Verification items for the finished model (mm, model axes). Face numbers are marked on the shaded views. A direction names the side the tool comes from. Round coordinates to 2 decimals unless told otherwise and drop trailing zeros. Loops run counter-clockwise (first coordinate to the right, second up) from the corner with the lowest first, then second, coordinate; pieces in that order, holes last. Notation, with made-up numbers: M 82,-17.5 L 137,-17.5 A22 cw 137,19.5 Z; hole C 29.5,15.5 d6. An arc over 180 degrees is marked long. Answer as CSV lines item,"result".
```python
from build123d import *

# Parameters (mm, degrees)
SKETCH3_R           = 1.7145000000000004
SKETCH3_R_2         = 1.7144999999999995
BOSS_EXTRUDE1_DEPTH = 3.175
BOSS_EXTRUDE2_DEPTH = 36.83
LPATTERN2_COUNT     = 2
LPATTERN2_PITCH     = 9.525
CUT_EXTRUDE1_DEPTH  = 54.24920844482103
FILLET1_R           = 3.175


with BuildPart() as part:
    # Sketch3 → Boss-Extrude1 (new body)
    with BuildSketch(Plane.XY):
        with BuildLine():
            ThreePointArc((23.718196461855243, 14.429078391112267), (20.955, 15.061802351494215), (18.191803538144754, 14.429078391112267))
            Line((18.191803538144754, 14.429078391112265), (-2.009608404339229, 4.6656054335111925))
            Line((-2.009608404339229, 4.6656054335111925), (-2.407325349839823, 4.473386263225946))
            ThreePointArc((-2.4073253498398226, 4.473386263225944), (-4.1812606420695575, -2.885040631096911), (3.3277025000445404, -3.83833245970139))
            Line((3.3277025000445413, -3.8383324597013875), (17.32713374877397, 5.9068077182607865))
            ThreePointArc((17.32713374877397, 5.9068077182607865), (20.955, 7.045177794406333), (24.58286625122603, 5.90680771826079))
            Line((24.58286625122603, 5.906807718260788), (38.58229749995545, -3.838332459701375))
            ThreePointArc((38.58229749995546, -3.8383324597013706), (46.09126064206956, -2.8850406310969055), (44.31732534983981, 4.4733862632259465))
            Line((44.31732534983981, 4.473386263225951), (43.91960840433945, 4.665605433511086))
            Line((43.91960840433945, 4.665605433511086), (23.718196461855243, 14.429078391112267))
        make_face()
        Circle(SKETCH3_R, mode=Mode.SUBTRACT)
        with Locations((41.91, 0)):
            Circle(SKETCH3_R_2, mode=Mode.SUBTRACT)
    boss_extrude1 = extrude(amount=BOSS_EXTRUDE1_DEPTH)

    # Sketch4 → Boss-Extrude2 (add)
    with BuildSketch(Plane(origin=(0, 15.239999999999998, 0), x_dir=(1, 0, 0), z_dir=(0, 1, 0))):
        Polygon((11.43, 0), (30.480000000000004, 2.33e-15), (30.48, 6.350000000000002), (11.43, 6.35), align=None)
    extrude(amount=-BOSS_EXTRUDE2_DEPTH)

    # LPattern2: Boss-Extrude1 ×2
    with Locations(*[(0, 0, -i * LPATTERN2_PITCH) for i in range(1, LPATTERN2_COUNT)]):
        add(boss_extrude1)

    # Sketch5 → Cut-Extrude1 (cut, through all)
    with BuildSketch(Plane.XY.offset(3.175)):
        with BuildLine():
            Line((36.195, 8.398958601029964), (23.718196461855243, 14.429078391112268))
            ThreePointArc((23.718196461855243, 14.429078391112268), (20.955, 15.061802351494219), (18.191803538144754, 14.429078391112267))
            Line((18.191803538144754, 14.429078391112267), (5.715000000000005, 8.39895860102995))
            Line((5.715000000000005, 8.39895860102995), (5.714999999999998, 15.239999999999984))
            Line((5.714999999999998, 15.239999999999984), (36.195, 15.239999999999998))
            Line((36.195, 15.239999999999998), (36.195, 8.398958601029964))
        make_face()
        with BuildLine():
            Line((30.480000000000004, 1.8017555908602794), (24.58286625122603, 5.906807718260787))
            ThreePointArc((24.58286625122603, 5.906807718260787), (20.955000000000002, 7.045177794406331), (17.327133748773974, 5.906807718260784))
            Line((17.327133748773974, 5.906807718260784), (11.430000000000003, 1.8017555908602725))
            Line((11.430000000000003, 1.8017555908602725), (11.430000000000026, -23.117342691118424))
            Line((11.430000000000026, -23.117342691118424), (30.480000000000004, -23.117342691118413))
            Line((30.480000000000004, -23.117342691118413), (30.480000000000004, 1.8017555908602794))
        make_face()
    extrude(amount=-CUT_EXTRUDE1_DEPTH, mode=Mode.SUBTRACT)

    # Fillet1
    fillet1_edges = [part.edges().sort_by_distance(p)[0] for p in [
        (30.480000000000004, 1.8017555908602794, -3.1750000000000016),
        (11.430000000000003, 1.8017555908602725, -3.175),
        (30.48, 11.161055038227271, -3.1750000000000016),
        (11.43, 11.16105503822726, -3.1749999999999994),
    ]]
    fillet(fillet1_edges, radius=FILLET1_R)


solid = part.part
```
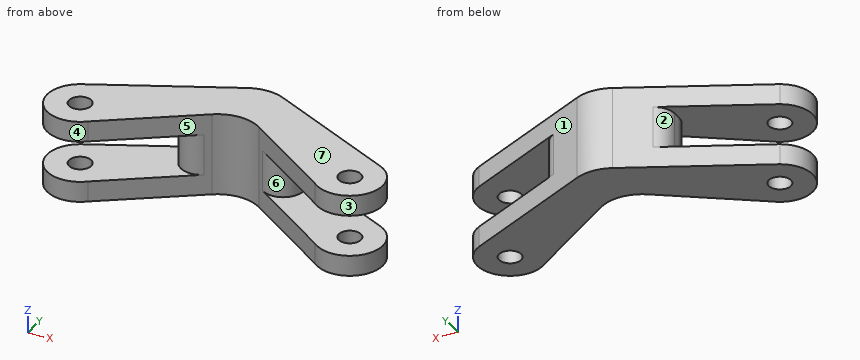
1) Section check B-B (z = -8.5). State how many separate pieces and enclosed holes the cut face has, plus the area to 3 significant figures.
Here are the results:
separate pieces,"1"
enclosed holes,"2"
area,"464 mm^2"
2) Material ranges on probe 1 along Z at (x, y) = (30.5, 5.75) (3 decimals); probe 2 along X at (y, z) = (6.5, -2.75); probe 3 along X at (y, z) = (9.75, -7.25), recorded low to high.
Here are the results:
probe 1,"z = -9.525 to -6.35, 0 to 3.175"
probe 2,"x = 11.75 to 18.38, 23.53 to 30.16"
probe 3,"x = 8.51 to 33.4"
3) Draft check along X on the marked faces 1, 2, 3 and 4. Enter one of: +X half, -X half, draft (parallel to the pull), parting line (faces both ways), or undercut.
Here are the results:
face 1,"+X half"
face 2,"-X half"
face 3,"undercut"
face 4,"undercut"
4) Go/stop test with flat-tipped pins: pin 1 (5.5 mm diameter, centred on x = 41.91, y = 0, fed in from -Z) (3 decimals); pin 2 (2 mm diameter, centred on x = 0, y = 0, fed in from +Z); pin 3 (1 mm diameter, centred on y = 8.5, z = -4.5, fed in from +X); pin 4 (5 mm diameter, centred on y = 8.5, z = 0, fed in from -X). Record where each tip stops, or that it passes through.
Here are the results:
pin 1,"stops at z = -9.525"
pin 2,"passes through"
pin 3,"stops at x = 30.48"
pin 4,"stops at x = 0.75"
5) Set-up check for the marked faces 5, 6 and 7: record each of +Z, -Z, +X, -X, +Y, -Y from which the full face is reachable in a straight line by a thin tool's end or side.
Here are the results:
face 5,"+Z, -Z, -Y"
face 6,"-Y"
face 7,"+Z, +X, -X, +Y, -Y"
6) Section check A-A (y = -2.5). Record the cut outline in (x, z) (3 decimals), plus the area to 3 significant figures.
Here are the results:
outline,"M -4.422,-9.525 L 5.25,-9.525 L 5.25,-6.35 L -4.422,-6.35 Z; M -4.422,0 L 5.25,0 L 5.25,3.175 L -4.422,3.175 Z; M 36.66,-9.525 L 46.332,-9.525 L 46.332,-6.35 L 36.66,-6.35 Z; M 36.66,0 L 46.332,0 L 46.332,3.175 L 36.66,3.175 Z"
area,"123 mm^2"
